Could you check a few things on this drawing? It's one solid part, dimensions in mm from its lowest x, y, z. A direction names the side the tool comes from. Give positions to 0.01 mm unless a question says otherwise; leave off trailing zeros. Loops run counter-clockwise (first coordinate to the right, second up) from the corner with the lowest first, then second, coordinate; pieces in that order, holes last. Notation, with made-up numbers: (70, 26) - (87, 26) arc R17 ccw to (87, 52) - close; hole circle Ø8 at (73, 74). An arc over 180 degrees is marked (long way). Write each question's results on one line, items separated by ' | '. Start each with the question number.
(1) Suppose I cut it at C-C (x = 37.5). Please give me the cut outline in (y, z).
(2) If we mould it in two halves opening along X, with no side actions, what happens to the marked faces 1, 2, 3 and 4? For each: released by +X, released by -X, zero draft, split by the parting line, or undercut.
(3) Suppose I cut it at A-A (z = 1.5). Please give me the cut outline in (x, y), and give its area (3 significant figures).
(4) On a 3-axis mill with a long thin cutter (end or side, diameter ignored), from which of +Z, -Z, +X, -X, +Y, -Y can I reach the whole of each face in a straight line? I mean the marked faces 5 and 6. Say none if no direction works.
(5) I need wall thicknesses on line 1 (X direction, y = 2, z = 5.75); line 2 (Z direction, x = 39, y = 0.75). Which ranges of each line are inside material? Lowest first, please.
(6) For pin 1 (3 mm diameter, centred on y = 1, z = 3, fed in from -X), with a flat end and sliding along its axis, tell me the tip position at first contact or that it passes through.
(7) Suppose I cut it at B-B (y = 4.75). Please give me the cut outline in (x, z), and give its area (3 significant figures).
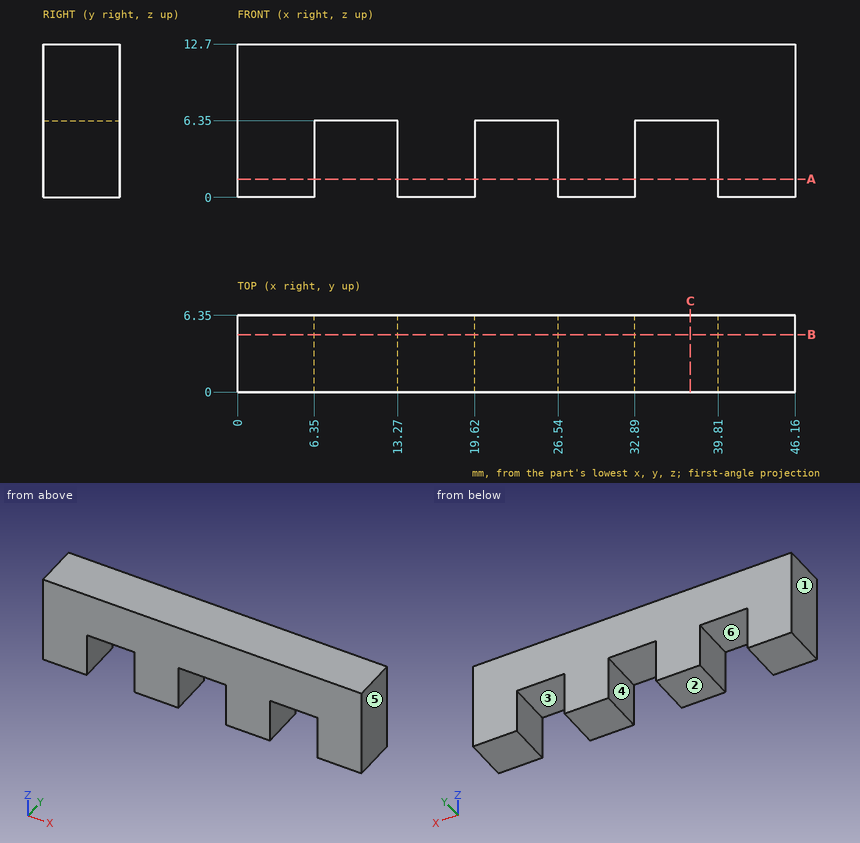
Output values:
1) outline: (0, 6.35) - (6.35, 6.35) - (6.35, 12.7) - (0, 12.7) - close
2) face 1: released by -X | face 2: zero draft | face 3: undercut | face 4: undercut
3) outline: (0, 0) - (6.35, 0) - (6.35, 6.35) - (0, 6.35) - close; (13.27, 0) - (19.62, 0) - (19.62, 6.35) - (13.27, 6.35) - close; (26.54, 0) - (32.89, 0) - (32.89, 6.35) - (26.54, 6.35) - close; (39.81, 0) - (46.16, 0) - (46.16, 6.35) - (39.81, 6.35) - close | area: 161 mm2
4) face 5: +Z, -Z, +X, +Y, -Y | face 6: -Z, +Y, -Y
5) line 1: 0 to 6.35, 13.27 to 19.62, 26.54 to 32.89, 39.81 to 46.16 | line 2: 6.35 to 12.7
6) pin 1: x = 0
7) outline: (0, 0) - (6.35, 0) - (6.35, 6.35) - (13.27, 6.35) - (13.27, 0) - (19.62, 0) - (19.62, 6.35) - (26.54, 6.35) - (26.54, 0) - (32.89, 0) - (32.89, 6.35) - (39.81, 6.35) - (39.81, 0) - (46.16, 0) - (46.16, 12.7) - (0, 12.7) - close | area: 454 mm2
